Verification items for the finished model (mm, model axes). A direction names the side the tool comes from. Round coordinates to 2 decimals unless told otherwise and drop trailing zeros. Write each loop counter-clockwise with the first axis right and the second up, starting at its lowest first coordinate (ties: lowest second). Pieces come first, ordered by that corner, then holes. Notation, with made-up numbers: M -11.5,-23 L 25.5,-23 A19 cw 25.5,-6 Z; hole C 21.5,-2 d7. An arc over 180 degrees is marked long. One line per question, with ' | ' between items.
from build123d import *

# Parameters (mm, degrees)
SKETCH1_W           = 172.72
SKETCH1_H           = 101.6
BOSS_EXTRUDE1_DEPTH = 5.85
SKETCH4_W           = 5.85
SKETCH4_H           = 33.866666666
SKETCH4_W_2         = 57.573333334
SKETCH4_H_2         = 5.85
SKETCH4_W_3         = 5.5
SKETCH4_H_3         = 4.5
CUT_EXTRUDE5_DEPTH  = 10
SKETCH5_R           = 9
SKETCH5_R_2         = 2.54
CUT_EXTRUDE10_DEPTH = 16
FILLET1_R           = 10
SKETCH6_R           = 2.85
CUT_EXTRUDE11_DEPTH = 10


with BuildPart() as part:
    # Sketch1 → Boss-Extrude1 (new body)
    with BuildSketch(Plane(origin=(0, 0, 0), x_dir=(1, 0, 0), z_dir=(0, 1, 0))):
        Rectangle(SKETCH1_W, SKETCH1_H)
    extrude(amount=BOSS_EXTRUDE1_DEPTH)

    # Sketch4 → Cut-Extrude5 (cut)
    with BuildSketch(Plane(origin=(0, 5.85, 0), x_dir=(1, 0, 0), z_dir=(0, 1, 0))):
        with Locations((-83.435, 0)):
            Rectangle(SKETCH4_W, SKETCH4_H)
        with Locations((0, -47.875)):
            Rectangle(SKETCH4_W_2, SKETCH4_H_2)
        with Locations((0, 47.875)):
            Rectangle(SKETCH4_W_2, SKETCH4_H_2)
        with Locations((63.61, 43)):
            Rectangle(SKETCH4_W_3, SKETCH4_H_3)
        with Locations((63.61, -43)):
            Rectangle(SKETCH4_W_3, SKETCH4_H_3)
        with Locations((63.61, -34)):
            Rectangle(SKETCH4_W_3, SKETCH4_H_3)
        with Locations((63.61, 34)):
            Rectangle(SKETCH4_W_3, SKETCH4_H_3)
    extrude(amount=-CUT_EXTRUDE5_DEPTH, mode=Mode.SUBTRACT)

    # Sketch5 → Cut-Extrude10 (cut)
    with BuildSketch(Plane(origin=(0, 0, 0), x_dir=(1, 0, 0), z_dir=(0, 1, 0))):
        with Locations(Location((-6.8720506, -0.189440326, 0), (0, 0, 90))):
            Circle(SKETCH5_R)
        with Locations(Location((-40.10375, -0.189440326, 0), (0, 0, 90))):
            Circle(SKETCH5_R)
        with Locations(Location((-63.676922318, 23.383731992, 0), (0, 0, 90))):
            Circle(SKETCH5_R_2)
        with Locations(Location((-16.530577682, 23.383731992, 0), (0, 0, 90))):
            Circle(SKETCH5_R_2)
        with Locations(Location((-63.676922318, -23.762612643, 0), (0, 0, 90))):
            Circle(SKETCH5_R_2)
        with Locations(Location((-16.530577682, -23.762612643, 0), (0, 0, 90))):
            Circle(SKETCH5_R_2)
        with Locations(Location((48.5139194, -0.189440326, 0), (0, 0, 90))):
            Circle(SKETCH5_R)
    extrude(amount=CUT_EXTRUDE10_DEPTH, mode=Mode.SUBTRACT)

    # Fillet1
    fillet1_edges = [part.edges().sort_by_distance(p)[0] for p in [
        (86.36, 2.925, 50.8),
        (86.36, 2.925, -50.8),
    ]]
    fillet(fillet1_edges, radius=FILLET1_R)

    # Sketch6 → Cut-Extrude11 (cut)
    with BuildSketch(Plane(origin=(0, 5.85, 0), x_dir=(1, 0, 0), z_dir=(0, 1, 0))):
        with Locations(Location((18.786666667, -34.95, 0), (0, 0, 270))):
            Circle(SKETCH6_R)
        with Locations(Location((18.786666667, 34.95, 0), (0, 0, 270))):
            Circle(SKETCH6_R)
    extrude(amount=-CUT_EXTRUDE11_DEPTH, mode=Mode.SUBTRACT)


solid = part.part
1. Mould release check, pull along Z, two halves, no side actions. Record for faces 1 (the face through (52, 3, 50.8)), 2 (the face through (-58, 3, -50.8)), 3 (the face through (66.36, 3, -43)), 4 (the face through (28.787, 3, 48)): pulls with the +Z half, pulls with the -Z half, needs draft (parallel to the pull), parting line crosses it, or undercut.
Results:
face 1: pulls with the +Z half | face 2: pulls with the -Z half | face 3: undercut | face 4: needs draft
2. Go/stop test with flat-tipped pins: P1, Ø1.5, axis at y = 4, z = 4.5, coming from the -X side; P2, Ø1.8, axis at x = 12.5, y = 2, coming from the +Z side. Record where each tip stops, or that it passes through.
Results:
P1: stops at x = -80.51 | P2: stops at z = 44.95
3. Section check A-A, the plane x = -45. Record the cut outline in (y, z), then the cut area to 3 significant figures.
Results:
outline: M 0,-50.8 L 5.85,-50.8 L 5.85,-7.36 L 0,-7.36 Z; M 0,7.74 L 5.85,7.74 L 5.85,50.8 L 0,50.8 Z | area: 506 mm2
4. Section check C-C, the plane x = 8. Record the cut outline in (y, z).
Results:
outline: M 0,-44.95 L 5.85,-44.95 L 5.85,44.95 L 0,44.95 Z
5. Tool access check on faces 5 (the face through (0, 3, -44.95)), 6 (the face through (64, 3, 40.75)), 7 (the face through (-80.51, 3, 0)). Record the directions out of +Z, -Z, +X, -X, +Y, -Y that give a thin tool (end or side, any length) a straight path to the whole face; none if there is none.
Results:
face 5: -Z, +Y, -Y | face 6: +Y, -Y | face 7: -X, +Y, -Y
6. Section check B-B, the plane y = 2.5. Count the separate pieces of the cut face and the enclosed holes in it, then the cut area to 3 significant figures.
Results:
separate pieces: 1 | enclosed holes: 13 | area: 15,600 mm2
7. Thickness scan on line 1 (X direction, y = 3.2, z = -36); line 2 (X direction, y = 4.6, z = 34.95); line 3 (X direction, y = 4.25, z = -5). Record the ranges inside material, lowest first.
Results:
line 1: x = -86.36 to 16.14, 21.44 to 60.86, 66.36 to 86.36 | line 2: x = -86.36 to 15.94, 21.64 to 60.86, 66.36 to 86.36 | line 3: x = -80.51 to -47.46, -32.75 to -14.23, 0.48 to 41.16, 55.87 to 86.36
